Source: CAD feature listing. Evaluate the final solid. Frame: model axes, mm. A direction names the side the tool comes from. Give positions to 0.01 mm unless a question says otherwise; leave off trailing zeros. Write each loop counter-clockwise with the first axis right and the second up, starting at its lowest first coordinate (ties: lowest second). Pieces come first, ordered by that corner, then holes.
```python
from build123d import *

# Parameters (mm, degrees)
SKETCH_1_R          = 14.5
EXTRUDE_1_DEPTH     = 157
EXTRUDE_2_DEPTH     = 21
SKETCH_3_R          = 4
CUT_EXTRUDE_1_DEPTH = 21
SKETCH_4_R          = 4
CUT_EXTRUDE_2_DEPTH = 80


with BuildPart() as part:
    # 草图1 → 凸台-拉伸1 (new body)
    with BuildSketch(Plane(origin=(0, 0, 0), x_dir=(0, 0, -1), z_dir=(1, 0, 0))):
        Circle(SKETCH_1_R)
    extrude(amount=EXTRUDE_1_DEPTH)

    # 草图2 → 凸台-拉伸2 (add)
    with BuildSketch(Plane(origin=(157, 0, 0), x_dir=(0, 0, -1), z_dir=(1, 0, 0))):
        with BuildLine():
            Line((-8, 7.549834435), (-8, -7.549834435))
            ThreePointArc((-8, -7.549834435), (0, -11), (8, -7.549834435))
            Line((8, -7.549834435), (8, 7.549834435))
            ThreePointArc((8, 7.549834435), (0, 11), (-8, 7.549834435))
        make_face()
    extrude(amount=EXTRUDE_2_DEPTH)

    # 草图3 → 切除-拉伸1 (cut)
    with BuildSketch(Plane.XY.offset(8)):
        with Locations((169, 0)):
            Circle(SKETCH_3_R)
    extrude(amount=-CUT_EXTRUDE_1_DEPTH, mode=Mode.SUBTRACT)

    # 草图4 → 切除-拉伸2 (cut)
    with BuildSketch(Plane.ZY):
        Circle(SKETCH_4_R)
    extrude(amount=-CUT_EXTRUDE_2_DEPTH, mode=Mode.SUBTRACT)


solid = part.part
```
1. Cut plane A-A, the plane y = 0. Return the cut outline in (x, z), then the cut area to 3 significant figures.
2. Contact query for flat-ended pins moving along their axis: P1, Ø16.5, axis at x = 171.5, y = 1.5, coming from the +Z side; P2, Ø5, axis at x = 139, z = -0.5, coming from the -Y side; P3, Ø5, axis at x = 148.5, y = -11.5, coming from the -Z side; P4, Ø3, axis at x = 126.5, z = 10.5, coming from the +Y side. Output: stop coordinate, or through.
3. Access query for faces 4 (the cylindrical face through (39.44, -3.905, -0.867)), 5 (the cylindrical face through (167, 11, 0)), 6 (the flat face through (165, 2, 8)). Directions: +Z, -Z, +X, -X, +Y, -Y. A direction counts if a zero-diameter tool reaches every point of the face in a straight line with its end or side. Return the directions, or none.
4. Cut plane C-C, the plane x = 169. Return the cut outline in (y, z), then the cut area to 3 significant figures.
5. Line query: L1, parallel to Y at x = 40.5, z = 0; L2, parallel to X at y = 0.5, z = -6.5; L3, parallel to Y at x = 169, z = -0.75. Output: solid intervals per line, ascending.
6. Cut plane D-D, the plane x = 133. Return the cut outline in (y, z), then the cut area to 3 significant figures.
7. Mould query, pull axis X, two halves, no side actions, for faces 1 (the cylindrical face through (172.815, 1.201, 0.112)), 2 (the flat face through (80, 0, 0)), 3 (the cylindrical face through (77.401, -12.864, -6.691)). Classes: +X half, -X half, draft (parallel to the pull), parting line (faces both ways), or undercut.
8. Cut plane B-B, the plane z = 0. Return the cut outline in (x, y), then the cut area to 3 significant figures.
Response values:
1. outline: (0, -14.5) - (157, -14.5) - (157, -8) - (165, -8) - (165, 8) - (157, 8) - (157, 14.5) - (0, 14.5) - (0, 4) - (80, 4) - (80, -4) - (0, -4) - close; (173, -8) - (178, -8) - (178, 8) - (173, 8) - close
1. area: 4,120 mm2
2. P1: stops at z = 8
2. P2: stops at y = -14.5
2. P3: stops at z = -11.37
2. P4: stops at y = 11.37
3. face 4: -X
3. face 5: +X, +Y
3. face 6: +Z, +X, +Y, -Y
4. outline: (-7.55, -8) - (-4, -8) - (-4, 8) - (-7.55, 8) arc R11 ccw to start; (4, -8) - (7.55, -8) arc R11 ccw to (7.55, 8) - (4, 8) - close
4. area: 190 mm2
5. L1: y = -14.5 to -4, 4 to 14.5
5. L2: x = 0 to 165.03, 172.97 to 178
5. L3: y = -10.97 to -4, 4 to 10.97
6. outline: circle Ø29 at (0, 0)
6. area: 661 mm2
7. face 1: undercut
7. face 2: -X half
7. face 3: draft
8. outline: (0, -14.5) - (157, -14.5) - (157, -11) - (178, -11) - (178, 11) - (157, 11) - (157, 14.5) - (0, 14.5) - (0, 4) - (80, 4) - (80, -4) - (0, -4) - close; hole circle Ø8 at (169, 0)
8. area: 4,320 mm2
